Design review of the part built by this model. Coordinates are the model's own, in mm. Coordinates: 2 decimals unless noted, no trailing zeros. Loops run counter-clockwise (first coordinate to the right, second up) from the corner with the lowest first, then second, coordinate; pieces in that order, holes last. Notation, with made-up numbers: (17.25, 35) -> (66.25, 35) arc R29 cw to (66.25, 55) -> close; hole circle Ø2 at (19.5, -28.5). An arc over 180 degrees is marked (long way). Use one line per item in the form item = value. Start each with the question number.
1. Consider section C-C (x = -22.5). State the section outline as (y, z) points, then the cut area to 3 significant figures.
2. Consider section B-B (x = -14). State the section outline as (y, z) points, then the cut area to 3 significant figures.
3. Wall thickness on line 1 (X direction, y = -9.5, z = 0.4); line 2 (Y direction, x = 10, z = 0.8); line 3 (Y direction, x = 1.5, z = 0.75): over which ranges is each line inside the solid? List them lowest first. Write a range as from..to.
4. For pin 1 (1.5 mm diameter, centred on x = 17, y = -23, fed in from +Z); pin 2 (1 mm diameter, centred on y = -22.5, z = 0.5, fed in from +X); pin 3 (0.8 mm diameter, centred on x = 10.5, z = 1.5, fed in from -Y), all flat-tipped, find the tip position at first contact; note any pin that passes through.
from build123d import *

# Parameters (mm, degrees)
F0_R     = 6.35
F1_DEPTH = 2.54
F2_R     = 1.26999


# Not quite as in the source:
# - a fillet or chamfer is up to 0.001 mm smaller than in the source, because OpenCascade refuses the exact size


with BuildPart() as f1:
    # F0 (on Top) → F1 (new body)
    with BuildSketch(Plane.XY):
        with BuildLine():
            Line((0.1342973504, 29.3290862039), (12.5991438484, 22.0549671115))
            ThreePointArc((12.5991438484, 22.0549671115), (12.7000000903, 21.997045204), (12.8005900541, 21.9386620893))
            Line((12.8005900541, 21.9386620893), (6.8682756911, 25.4))
            Line((6.8682756911, 25.4), (0.1342973504, 29.3290862039))
        make_face()
        with BuildLine():
            ThreePointArc((-12.5991438484, 22.0549671115), (0, 25.4), (12.5991438484, 22.0549671115))
            Line((12.5991438484, 22.0549671115), (0.1342973504, 29.3290862039))
            Line((0.1342973504, 29.3290862039), (-6.7436197563, 25.4))
            Line((-6.7436197563, 25.4), (-12.5991438484, 22.0549671115))
        make_face()
        Polygon((-18.5629074106, 18.6481012287), (-12.5991438484, 22.0549671115), (-6.7436197563, 25.4), (-14.6646968374, 25.4), align=None)
        with BuildLine():
            ThreePointArc((-25.3997337218, 0.1163050384), (-21.9386621638, 12.8005899263), (-12.5991438484, 22.0549671115))
            Line((-12.5991438484, 22.0549671115), (-18.5629074106, 18.6481012287))
            Line((-18.5629074106, 18.6481012287), (-25.3325850472, 14.780848019))
            Line((-25.3325850472, 14.780848019), (-25.3688551343, 6.8598539776))
            Line((-25.3688551343, 6.8598539776), (-25.3997337218, 0.1163050384))
        make_face()
        with BuildLine():
            Line((18.625235378, 18.5401460224), (12.8005900541, 21.9386620893))
            ThreePointArc((12.8005900541, 21.9386620893), (12.8993470878, 21.8807414113), (12.9978420445, 21.822376181))
            Line((12.9978420446, 21.822376181), (25.4668823975, 14.5482381848))
            Line((25.4668823975, 14.5482381848), (18.625235378, 18.5401460224))
        make_face()
        Polygon((6.8682756911, 25.4), (12.8005900541, 21.9386620893), (18.625235378, 18.5401460224), (14.6646968374, 25.4), align=None)
        with BuildLine():
            Line((25.4668823975, 14.5482381848), (12.9978420446, 21.822376181))
            ThreePointArc((12.9978420445, 21.822376181), (22.0828574683, 12.550195458), (25.4, 0))
            ThreePointArc((25.4, 0), (25.3999334305, -0.0581525957), (25.3997337225, -0.1163048866))
            Line((25.3997337225, -0.1163048866), (25.4002662804, 0))
            Line((25.4002662804, 0), (25.4311831017, 6.7518987713))
            Line((25.4311831017, 6.7518987713), (25.4668823975, 14.5482381848))
        make_face()
        Polygon((-25.4002662804, 0), (-25.3997337218, 0.1163050384), (-25.3688551343, 6.8598539776), (-29.3293936748, 0), (-25.4311831017, -6.7518987713), align=None)
        with BuildLine():
            ThreePointArc((-21.9970455091, -12.6999995618), (-24.5495027703, -6.5178151043), (-25.3997337218, 0.1163050384))
            Line((-25.3997337218, 0.1163050384), (-25.4002662804, 0))
            Line((-25.4002662804, 0), (-25.4311831017, -6.7518987713))
            Line((-25.4311831017, -6.7518987713), (-21.9970455091, -12.6999995618))
        make_face()
        with BuildLine():
            ThreePointArc((-12.800589874, -21.9386621944), (-18.0015854544, -17.9193448856), (-21.9970455091, -12.6999995618))
            Line((-21.9970455091, -12.6999995618), (-18.625235378, -18.5401460224))
            Line((-18.625235378, -18.5401460224), (-12.800589874, -21.9386621944))
        make_face()
        Polygon((-18.625235378, -18.5401460224), (-21.9970455091, -12.6999995618), (-25.4311831017, -6.7518987713), (-25.4668823975, -14.5482381848), align=None)
        with BuildLine():
            Line((25.3688551343, -6.8598539776), (25.3997337225, -0.1163048866))
            ThreePointArc((25.3997337225, -0.1163048866), (22.6367712709, -11.5211365077), (15.0421744156, -20.4668754052))
            Line((15.0421744156, -20.4668754052), (18.6118299226, -18.4944410973))
            Line((18.6118299226, -18.4944410973), (25.3325850472, -14.780848019))
            Line((25.3325850472, -14.780848019), (25.3688551343, -6.8598539776))
        make_face()
        Polygon((25.4002662804, 0), (25.3997337225, -0.1163048866), (25.3688551343, -6.8598539776), (29.3293936748, 0), (25.4311831017, 6.7518987713), align=None)
        with BuildLine():
            ThreePointArc((-12.1717221157, -22.2937027149), (-12.4874178664, -22.1184175526), (-12.800589874, -21.9386621944))
            Line((-12.800589874, -21.9386621944), (-18.625235378, -18.5401460224))
            Line((-18.625235378, -18.5401460224), (-14.6646968374, -25.4))
            Line((-14.6646968374, -25.4), (-6.9223574365, -25.2573419592))
            Line((-6.9223574365, -25.2573419592), (-12.1717221157, -22.2937027149))
        make_face()
        with BuildLine():
            Line((18.6118299226, -18.4944410973), (15.0421744156, -20.4668754052))
            ThreePointArc((15.0421744156, -20.4668754052), (12.4565037471, -22.1358423015), (9.6879678482, -23.4798483592))
            Line((9.6879678482, -23.4798483592), (6.7447131478, -25.1612151536))
            Line((6.7447131478, -25.1612151536), (14.6657902289, -25.1612151536))
            Line((14.6657902289, -25.1612151536), (18.6118299226, -18.4944410973))
        make_face()
        with BuildLine():
            ThreePointArc((9.6879678482, -23.4798483592), (-1.3762246139, -25.3626892465), (-12.1717221157, -22.2937027149))
            Line((-12.1717221157, -22.2937027149), (-6.9223574365, -25.2573419592))
            Line((-6.9223574365, -25.2573419592), (-0.1332039589, -29.0903013575))
            Line((-0.1332039589, -29.0903013575), (6.7447131478, -25.1612151536))
            Line((6.7447131478, -25.1612151536), (9.6879678482, -23.4798483592))
        make_face()
        with BuildLine():
            Line((12.9978420446, 21.822376181), (12.5991438484, 22.0549671115))
            ThreePointArc((12.5991438484, 22.0549671115), (0, 25.4), (-12.5991438484, 22.0549671115))
            ThreePointArc((-12.5991438484, 22.0549671115), (-21.9386621638, 12.8005899263), (-25.3997337218, 0.1163050384))
            ThreePointArc((-25.3997337218, 0.1163050384), (-24.5495027703, -6.5178151043), (-21.9970455091, -12.6999995618))
            ThreePointArc((-21.9970455091, -12.6999995618), (-18.0015854544, -17.9193448856), (-12.800589874, -21.9386621944))
            Line((-12.800589874, -21.9386621944), (-12.1717221157, -22.2937027149))
            ThreePointArc((-12.1717221157, -22.2937027149), (-1.3762246139, -25.3626892465), (9.6879678482, -23.4798483592))
            Line((9.6879678482, -23.4798483592), (12.6002372398, -21.8161822651))
            Line((12.6002372398, -21.8161822651), (15.0421744156, -20.4668754052))
            ThreePointArc((15.0421744156, -20.4668754052), (22.6367712709, -11.5211365077), (25.3997337225, -0.1163048866))
            ThreePointArc((25.3997337225, -0.1163048866), (25.3999334305, -0.0581525957), (25.4, 0))
            ThreePointArc((25.4, 0), (22.0828574683, 12.550195458), (12.9978420445, 21.822376181))
        make_face()
        Circle(F0_R, mode=Mode.SUBTRACT)
        with BuildLine():
            ThreePointArc((9.6879678482, -23.4798483592), (12.4565037471, -22.1358423015), (15.0421744156, -20.4668754052))
            Line((15.0421744156, -20.4668754052), (12.6002372398, -21.8161822651))
            Line((12.6002372398, -21.8161822651), (9.6879678482, -23.4798483592))
        make_face()
    extrude(amount=F1_DEPTH)

    # F2 (radius 1.27 in the source; OpenCascade refuses exactly that, so slightly less here)
    f2_edges = [f1.edges().sort_by_distance(p)[0] for p in [
        (-6.35, 0, 2.54),
        (-6.35, 0, 0),
    ]]
    fillet(f2_edges, radius=F2_R)


solid = f1.part
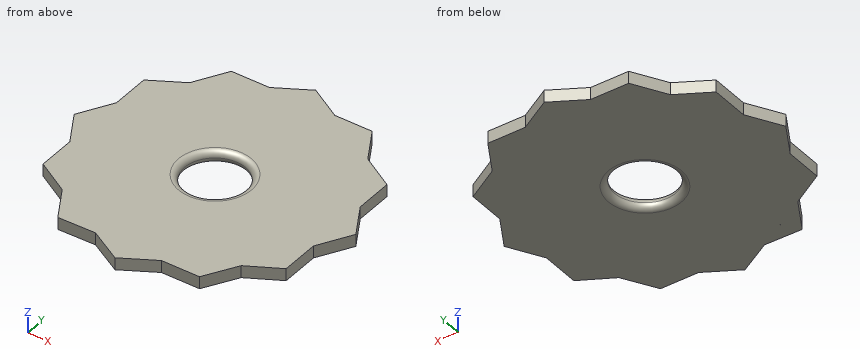
Geometry check:
q1.outline = (-16.28, 0) -> (16.4, 0) -> (16.4, 2.54) -> (-16.28, 2.54) -> close
q1.area = 83.0 mm²
q2.outline = (-25.39, 0) -> (25.4, 0) -> (25.4, 2.54) -> (-25.39, 2.54) -> close
q2.area = 129 mm²
q3.line_1 = -25.44..25.36
q3.line_2 = -25.16..25.4
q3.line_3 = -28.16..-6.28, 6.28..28.53
q4.pin_1 = through
q4.pin_2 = 16.54
q4.pin_3 = -25.16
